Read the model definition and answer for the solid it produces. Units are mm, in the model's axes. Give positions to 0.01 mm unless a question says otherwise; leave off trailing zeros. Loops run counter-clockwise (first coordinate to the right, second up) from the corner with the lowest first, then second, coordinate; pieces in that order, holes last. Notation, with made-up numbers: (-11, 41.25) - (2, 41.25) arc R22 ccw to (2, 56.25) - close; hole circle Ø11 at (-23, 59.5). An arc over 180 degrees is marked (long way). Write item = value, one per line.
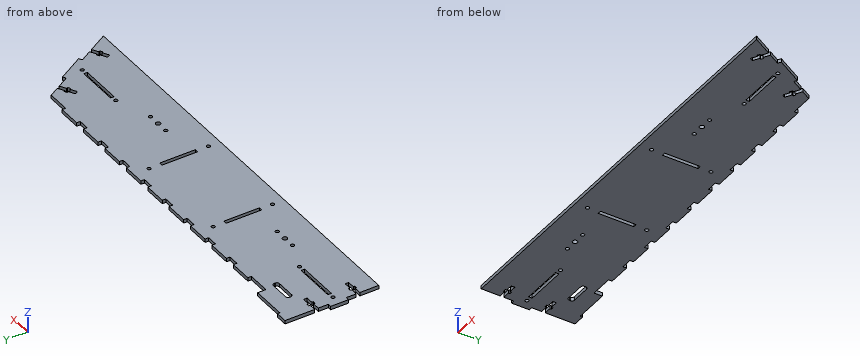
```python
from build123d import *

# Parameters (mm, degrees)
SKETCH_1_R             = 2
SKETCH_1_R_2           = 1.5
EXTRUDE_1_DEPTH        = 3
SKETCH_2_W             = 19
SKETCH_2_H             = 3
EXTRUDE_2_DEPTH        = 3
PATTERN_LINEAR_1_COUNT = 9
PATTERN_LINEAR_1_PITCH = 28
SKETCH_3_W             = 3
SKETCH_3_H             = 30
CUT_EXTRUDE_1_DEPTH    = 3
SKETCH_4_W             = 35
SKETCH_4_H             = 3
CUT_EXTRUDE_2_DEPTH    = 3
SKETCH_5_R             = 1.5
CUT_EXTRUDE_3_DEPTH    = 3
CUT_EXTRUDE_4_DEPTH    = 3
CUT_EXTRUDE_5_DEPTH    = 3
SKETCH_8_W             = 39
SKETCH_8_H             = 3
EXTRUDE_3_DEPTH        = 9
SKETCH_9_W             = 29
SKETCH_9_H             = 3
CUT_EXTRUDE_6_DEPTH    = 2
SKETCH_11_W            = 3
SKETCH_11_H            = 25
EXTRUDE_5_DEPTH        = 3
SKETCH_12_W            = 3
SKETCH_12_H            = 15
EXTRUDE_6_DEPTH        = 3
SKETCH_13_W            = 20
SKETCH_13_H            = 5
CUT_EXTRUDE_7_DEPTH    = 3
FILLET_1_R             = 2


with BuildPart() as part:
    # Эскиз1 → Бобышка-Вытянуть1 (new body)
    with BuildSketch(Plane.XY):
        Polygon((320, 70), (360.414518843, 0), (0, 0), (0, 70), align=None)
        with Locations((84, 25)):
            Circle(SKETCH_1_R, mode=Mode.SUBTRACT)
        with Locations((250, 25)):
            Circle(SKETCH_1_R, mode=Mode.SUBTRACT)
        with Locations((94, 25)):
            Circle(SKETCH_1_R_2, mode=Mode.SUBTRACT)
        with Locations((74, 25)):
            Circle(SKETCH_1_R_2, mode=Mode.SUBTRACT)
        with Locations((240, 25)):
            Circle(SKETCH_1_R_2, mode=Mode.SUBTRACT)
        with Locations((260, 25)):
            Circle(SKETCH_1_R_2, mode=Mode.SUBTRACT)
    extrude(amount=EXTRUDE_1_DEPTH)

    # Эскиз2 → Бобышка-Вытянуть2 (add)
    with BuildSketch(Plane(origin=(0, 70, 0), x_dir=(1, 0, 0), z_dir=(0, 1, 0))):
        with Locations((291.5, -1.5)):
            Rectangle(SKETCH_2_W, SKETCH_2_H)
    extrude_2 = extrude(amount=EXTRUDE_2_DEPTH)

    # Линейный массив1: Бобышка-Вытянуть2 ×9
    with Locations(*[(-i * PATTERN_LINEAR_1_PITCH, 0, 0) for i in range(1, PATTERN_LINEAR_1_COUNT)]):
        add(extrude_2)

    # Эскиз3 → Вырез-Вытянуть1 (cut)
    with BuildSketch(Plane.XY.offset(3)):
        with Locations((207.5, 35)):
            Rectangle(SKETCH_3_W, SKETCH_3_H)
        with Locations((123.5, 35)):
            Rectangle(SKETCH_3_W, SKETCH_3_H)
    extrude(amount=-CUT_EXTRUDE_1_DEPTH, mode=Mode.SUBTRACT)

    # Эскиз4 → Вырез-Вытянуть2 (cut)
    with BuildSketch(Plane.XY.offset(3)):
        with Locations((311.841234018, 35)):
            Rectangle(SKETCH_4_W, SKETCH_4_H)
        with Locations((27.5, 35)):
            Rectangle(SKETCH_4_W, SKETCH_4_H)
    extrude(amount=-CUT_EXTRUDE_2_DEPTH, mode=Mode.SUBTRACT)

    # Эскиз5 → Вырез-Вытянуть3 (cut)
    with BuildSketch(Plane.XY.offset(3)):
        with Locations((5.5, 35)):
            Circle(SKETCH_5_R)
        with Locations((49.5, 35)):
            Circle(SKETCH_5_R)
        with Locations((123.5, 60)):
            Circle(SKETCH_5_R)
        with Locations((123.5, 10)):
            Circle(SKETCH_5_R)
        with Locations((207.5, 60)):
            Circle(SKETCH_5_R)
        with Locations((207.5, 10)):
            Circle(SKETCH_5_R)
        with Locations((289.841234018, 35)):
            Circle(SKETCH_5_R)
        with Locations((333.841234018, 35)):
            Circle(SKETCH_5_R)
    extrude(amount=-CUT_EXTRUDE_3_DEPTH, mode=Mode.SUBTRACT)

    # Эскиз6 → Вырез-Вытянуть4 (cut)
    with BuildSketch(Plane.XY.offset(3)):
        Polygon((0, 54), (6, 54), (6, 55.25), (8.5, 55.25), (8.5, 54), (14.5, 54), (14.5, 51), (8.5, 51), (8.5, 49.75), (6, 49.75), (6, 51), (0, 51), align=None)
        Polygon((0, 19), (6, 19), (6, 20.25), (8.5, 20.25), (8.5, 19), (14.5, 19), (14.5, 16), (8.5, 16), (8.5, 14.75), (6, 14.75), (6, 16), (0, 16), align=None)
    extrude(amount=-CUT_EXTRUDE_4_DEPTH, mode=Mode.SUBTRACT)

    # Эскиз7 → Вырез-Вытянуть5 (cut)
    with BuildSketch(Plane.XY.offset(3)):
        Polygon((324.664518843, 61.920816371), (319.468366421, 58.920816371), (318.843366421, 60.003348125), (316.678302911, 58.753348125), (317.303302911, 57.670816371), (312.107150488, 54.670816371), (313.607150488, 52.072740159), (318.803302911, 55.072740159), (319.428302911, 53.990208405), (321.593366421, 55.240208405), (320.968366421, 56.322740159), (326.164518843, 59.322740159), align=None)
        Polygon((349.664518843, 18.619546181), (344.468366421, 15.619546181), (343.843366421, 16.702077936), (341.678302911, 15.452077936), (342.303302911, 14.369546181), (337.107150488, 11.369546181), (338.607150488, 8.77146997), (343.803302911, 11.77146997), (344.428302911, 10.688938215), (346.593366421, 11.938938215), (345.968366421, 13.02146997), (351.164518843, 16.02146997), align=None)
    extrude(amount=-CUT_EXTRUDE_5_DEPTH, mode=Mode.SUBTRACT)

    # Эскиз8 → Бобышка-Вытянуть3 (add)
    with BuildSketch(Plane(origin=(0, 70, 0), x_dir=(1, 0, 0), z_dir=(0, 1, 0))):
        with Locations((19.5, -1.5)):
            Rectangle(SKETCH_8_W, SKETCH_8_H)
    extrude(amount=EXTRUDE_3_DEPTH)

    # Эскиз9 → Вырез-Вытянуть6 (cut)
    with BuildSketch(Plane(origin=(0, 79, 0), x_dir=(1, 0, 0), z_dir=(0, 1, 0))):
        with Locations((24.5, -1.5)):
            Rectangle(SKETCH_9_W, SKETCH_9_H)
    extrude(amount=-CUT_EXTRUDE_6_DEPTH, mode=Mode.SUBTRACT)

    # Эскиз11 → Бобышка-Вытянуть5 (add)
    with BuildSketch(Plane(origin=(270.310889132, 156.064064606, 0), x_dir=(0, 0, -1), z_dir=(0.8660254037844416, 0.4999999999999949, 0))):
        with Locations((-1.5, -135.207259422)):
            Rectangle(SKETCH_11_W, SKETCH_11_H)
    extrude(amount=EXTRUDE_5_DEPTH)

    # Эскиз12 → Бобышка-Вытянуть6 (add)
    with BuildSketch(Plane.ZY):
        with Locations((1.5, 35)):
            Rectangle(SKETCH_12_W, SKETCH_12_H)
    extrude(amount=EXTRUDE_6_DEPTH)

    # Эскиз13 → Вырез-Вытянуть7 (cut)
    with BuildSketch(Plane.XY.offset(3)):
        with Locations((32.07564967, 60.49517076)):
            Rectangle(SKETCH_13_W, SKETCH_13_H)
    extrude(amount=-CUT_EXTRUDE_7_DEPTH, mode=Mode.SUBTRACT)

    # Скругление1
    fillet_1_edges = [part.edges().sort_by_distance(p)[0] for p in [
        (22.07564967, 57.99517076, 1.5),
        (22.07564967, 62.99517076, 1.5),
        (42.07564967, 62.99517076, 1.5),
        (42.07564967, 57.99517076, 1.5),
    ]]
    fillet(fillet_1_edges, radius=FILLET_1_R)


solid = part.part
```
1) Find the intervals of material crossed by probe 1 along X at (y, z) = (46.5, 2.7); probe 2 along X at (y, z) = (49.5, 2.6); probe 3 along Y at (x, z) = (74, 1.9), in increasing order.
Output:
probe_1 = 0 to 122, 125 to 206, 209 to 337.03
probe_2 = 0 to 122, 125 to 206, 209 to 335.3
probe_3 = 0 to 23.5, 26.5 to 73
2) Each of these flat-tipped pins is pushed along its axis until it touches: P1, Ø0.9, axis at y = 71, z = 1.5, coming from the +X side; P2, Ø1.5, axis at x = 309, z = 1.5, coming from the +Y side; P3, Ø0.9, axis at x = -1, z = 1, coming from the +Y side. Where does it stop, or does it pass through?
Output:
P1 = 301
P2 = 70
P3 = 42.5
3) A cutting plane is placed at B-B on z = 2.1. Give the number of separate pieces and of enclosed holes in the cut face, then the cut area to 3 significant figures.
Output:
separate_pieces = 1
enclosed_holes = 19
area = 23,900 mm²
4) A cutting plane is placed at A-A on x = 177. Determine the outline of the cut face in (y, z), then the cut area to 3 significant figures.
Output:
outline = (0, 0) - (73, 0) - (73, 3) - (0, 3) - close
area = 219 mm²
